Input: part model. Units: mm. Frame: model coordinates. Face numbers are marked on the shaded views. A direction names the side the tool comes from. Give positions to 0.01 mm unless a question says otherwise; leave off trailing zeros. Loops run counter-clockwise (first coordinate to the right, second up) from the corner with the lowest first, then second, coordinate; pieces in that order, holes last. Notation, with made-up numbers: M 54.25,-27 L 61.25,-27 A9 ccw 61.25,-20 Z; hole C 6,-9 d2. An arc over 180 degrees is marked long. Answer as a JSON object with one key per item and string values. Group by question number.
```python
from build123d import *

# Parameters (mm, degrees)
SKETCH_1_R      = 1.5
EXTRUDE_2_DEPTH = 6


with BuildPart() as part:
    # 草图1 → 凸台-拉伸2 (new body)
    with BuildSketch(Plane.XY):
        with BuildLine():
            Line((24, 3.84), (10.710014006, 3.84))
            ThreePointArc((10.710014006, 3.84), (7.476263419, 4.377291236), (4.590006002, 5.931428571))
            ThreePointArc((4.590006002, 5.931428571), (-7.5, 0), (4.590006002, -5.931428571))
            ThreePointArc((4.590006002, -5.931428571), (7.476263419, -4.377291236), (10.710014006, -3.84))
            Line((10.710014006, -3.84), (24, -3.84))
            ThreePointArc((24, -3.84), (27.84, 0), (24, 3.84))
        make_face()
        Circle(SKETCH_1_R, mode=Mode.SUBTRACT)
        with Locations((20, 0)):
            Circle(SKETCH_1_R, mode=Mode.SUBTRACT)
        with Locations((24, 0)):
            Circle(SKETCH_1_R, mode=Mode.SUBTRACT)
    extrude(amount=EXTRUDE_2_DEPTH)


solid = part.part
```
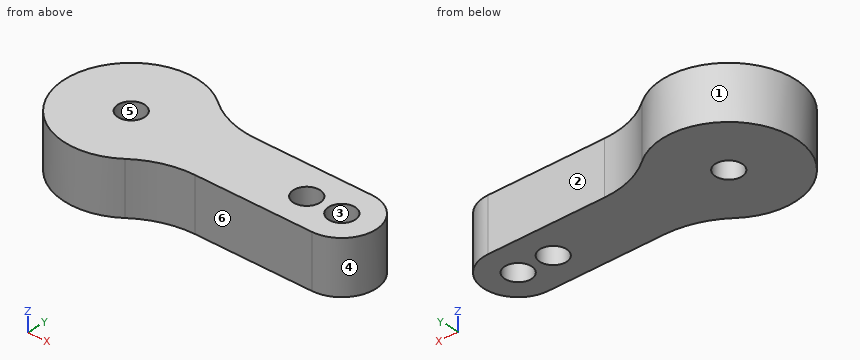
1. Section B-B (y = 0). Output: boundary loops of the cut face in (x, z), then the cut area to 3 significant figures.
2. Section D-D (x = 24.5). Output: boundary loops of the cut face in (y, z).
3. Section C-C (z = 2). Output: boundary loops of the cut face in (x, y).
4. Material intervals for L1, parallel to Y at x = 24, z = 4.65; L2, parallel to Y at x = 0, z = 1.3; L3, parallel to X at y = -1.25, z = 5.15, sorted ascending.
5. First-contact query: P1, Ø3, axis at y = 4, z = 3, coming from the +X side; P2, Ø1.5, axis at y = -3.5, z = 2.5, coming from the +X side; P3, Ø1.8, axis at x = 17.5, z = 3.5, coming from the -Y side. Flat tips, straight axial feed; report the tip coordinate or a pass-through.
6. Reachability of the marked faces 5 and 6 from +Z, -Z, +X, -X, +Y, -Y: full face, straight path, thin tool, end or side. Return the list, or none.
7. Section A-A (x = 0). Output: boundary loops of the cut face in (y, z), then the cut area to 3 significant figures.
8. Mould query, pull axis X, two halves, no side actions, for the marked faces 1, 2, 3 and 4. Classes: pulls with the +X half, pulls with the -X half, needs draft (parallel to the pull), parting line crosses it, or undercut.
Geometry results:
{
 "1": {"outline": "M -7.5,0 L -1.5,0 L -1.5,6 L -7.5,6 Z; M 1.5,0 L 18.5,0 L 18.5,6 L 1.5,6 Z; M 21.5,0 L 22.5,0 L 22.5,6 L 21.5,6 Z; M 25.5,0 L 27.84,0 L 27.84,6 L 25.5,6 Z", "area": "158 mm2"},
 "2": {"outline": "M -3.81,0 L -1.41,0 L -1.41,6 L -3.81,6 Z; M 1.41,0 L 3.81,0 L 3.81,6 L 1.41,6 Z"},
 "3": {"outline": "M 4.59,-5.93 A10 cw 10.71,-3.84 L 24,-3.84 A3.84 ccw 24,3.84 L 10.71,3.84 A10 cw 4.59,5.93 A7.5 ccw long Z; hole C 0,0 d3; hole C 20,0 d3; hole C 24,0 d3"},
 "4": {"L1": "-3.84 to -1.5, 1.5 to 3.84", "L2": "-7.5 to -1.5, 1.5 to 7.5", "L3": "-7.4 to -0.83, 0.83 to 19.17, 20.83 to 23.17, 24.83 to 27.63"},
 "5": {"P1": "x = 26.91", "P2": "x = 26.68", "P3": "y = -3.84"},
 "6": {"face 5": "+Z, -Z", "face 6": "+Z, -Z, +X, -Y"},
 "7": {"outline": "M -7.5,0 L -1.5,0 L -1.5,6 L -7.5,6 Z; M 1.5,0 L 7.5,0 L 7.5,6 L 1.5,6 Z", "area": "72.0 mm2"},
 "8": {"face 1": "parting line crosses it", "face 2": "needs draft", "face 3": "undercut", "face 4": "pulls with the +X half"}
}
